from build123d import *

# Parameters (mm, degrees)
F0_R     = 4.5
F1_DEPTH = 8
F0_R_2   = 29
F0_R_3   = 27
F2_DEPTH = 4


with BuildPart() as f1:
    # F0 (on Front) → F1 (new body)
    with BuildSketch(Plane.XZ):
        Circle(F0_R)
    extrude(amount=F1_DEPTH)

    # F0 (on Front) → F2 (join)
    with BuildSketch(Plane.XZ):
        Circle(F0_R_2)
        Circle(F0_R_3, mode=Mode.SUBTRACT)
        Circle(F0_R_3)
        with BuildLine():
            ThreePointArc((4.3516162867, -22.646052221), (-0.1431680004, -25.9977219705), (-4.4156935051, -22.3669780097))
            Line((-4.4156935051, -22.3669780097), (0, -7.75))
            Line((0, -7.75), (4.3516162867, -22.646052221))
        make_face(mode=Mode.SUBTRACT)
        with BuildLine():
            ThreePointArc((-19.4040272759, -5.6313106345), (-17.9803864059, -4.3071155471), (-16.1592835692, -3.626064584))
            Line((-16.1592835692, -3.626064584), (-9.3891987076, -2.5182325158))
            ThreePointArc((-9.3891987076, -2.5182325158), (-7.4460025695, -2.583307283), (-5.6745435039, -3.3846678354))
            ThreePointArc((-5.6745435039, -3.3846678354), (-4.4349924254, -4.4349924254), (-3.3846678354, -5.6745435039))
            ThreePointArc((-3.3846678354, -5.6745435039), (-2.583307283, -7.4460025695), (-2.5182325158, -9.3891987076))
            Line((-2.5182325158, -9.3891987076), (-3.626064584, -16.1592835692))
            ThreePointArc((-3.626064584, -16.1592835692), (-4.3071155471, -17.9803864059), (-5.6313106345, -19.4040272759))
            ThreePointArc((-5.6313106345, -19.4040272759), (-18.3847763109, -18.3847763109), (-19.4040272759, -5.6313106345))
        make_face(mode=Mode.SUBTRACT)
        with BuildLine():
            Line((3.6418333236, -16.2556480886), (2.5157025337, -9.3737377061))
            ThreePointArc((2.5157025337, -9.3737377061), (2.5903516211, -7.3902488103), (3.4308544392, -5.5920953967))
            ThreePointArc((3.4308544392, -5.5920953967), (4.5023744658, -4.3693333532), (5.760194673, -3.3391923392))
            ThreePointArc((5.760194673, -3.3391923392), (7.5038582162, -2.5767129031), (9.4061289224, -2.5210029146))
            Line((9.4061289224, -2.5210029146), (16.060956923, -3.6099747692))
            ThreePointArc((16.060956923, -3.6099747692), (17.8462537904, -4.2691049062), (19.2559417587, -5.5475873168))
            ThreePointArc((19.2559417587, -5.5475873168), (18.450217913, -18.3171768004), (5.7146063745, -19.5483572234))
            ThreePointArc((5.7146063745, -19.5483572234), (4.344802068, -18.1118904301), (3.6418333236, -16.2556480886))
        make_face(mode=Mode.SUBTRACT)
        with BuildLine():
            ThreePointArc((-22.3669780097, -4.4156935051), (-26, 0), (-22.3669780097, 4.4156935051))
            Line((-22.3669780097, 4.4156935051), (-7.75, 0))
            Line((-7.75, 0), (-22.3669780097, -4.4156935051))
        make_face(mode=Mode.SUBTRACT)
        with BuildLine():
            Line((-9.3891987076, 2.5182325158), (-16.1592835692, 3.626064584))
            ThreePointArc((-16.1592835692, 3.626064584), (-17.9803864059, 4.3071155471), (-19.4040272759, 5.6313106345))
            ThreePointArc((-19.4040272759, 5.6313106345), (-18.3847763109, 18.3847763109), (-5.6313106345, 19.4040272759))
            ThreePointArc((-5.6313106345, 19.4040272759), (-4.3071155471, 17.9803864059), (-3.626064584, 16.1592835692))
            Line((-3.626064584, 16.1592835692), (-2.5182325158, 9.3891987076))
            ThreePointArc((-2.5182325158, 9.3891987076), (-2.583307283, 7.4460025695), (-3.3846678354, 5.6745435039))
            ThreePointArc((-3.3846678354, 5.6745435039), (-4.4349924254, 4.4349924254), (-5.6745435039, 3.3846678354))
            ThreePointArc((-5.6745435039, 3.3846678354), (-7.4460025695, 2.583307283), (-9.3891987076, 2.5182325158))
        make_face(mode=Mode.SUBTRACT)
        Circle(F0_R, mode=Mode.SUBTRACT)
        with BuildLine():
            Line((16.1592835692, 3.626064584), (9.3891987076, 2.5182325158))
            ThreePointArc((9.3891987076, 2.5182325158), (7.4460025695, 2.583307283), (5.6745435039, 3.3846678354))
            ThreePointArc((5.6745435039, 3.3846678354), (4.4349924254, 4.4349924254), (3.3846678354, 5.6745435039))
            ThreePointArc((3.3846678354, 5.6745435039), (2.583307283, 7.4460025695), (2.5182325158, 9.3891987076))
            Line((2.5182325158, 9.3891987076), (3.626064584, 16.1592835692))
            ThreePointArc((3.626064584, 16.1592835692), (4.3071155471, 17.9803864059), (5.6313106345, 19.4040272759))
            ThreePointArc((5.6313106345, 19.4040272759), (18.3847763109, 18.3847763109), (19.4040272759, 5.6313106345))
            ThreePointArc((19.4040272759, 5.6313106345), (17.9803864059, 4.3071155471), (16.1592835692, 3.626064584))
        make_face(mode=Mode.SUBTRACT)
        with BuildLine():
            ThreePointArc((22.3669780097, 4.4156935051), (26, 0), (22.3669780097, -4.4156935051))
            Line((22.3669780097, -4.4156935051), (7.75, 0))
            Line((7.75, 0), (14.262410288, 1.9673565762))
            Line((14.262410288, 1.9673565762), (22.3669780097, 4.4156935051))
        make_face(mode=Mode.SUBTRACT)
        with BuildLine():
            ThreePointArc((-4.4156935051, 22.3669780097), (0, 26), (4.4156935051, 22.3669780097))
            Line((4.4156935051, 22.3669780097), (0, 7.75))
            Line((0, 7.75), (-4.4156935051, 22.3669780097))
        make_face(mode=Mode.SUBTRACT)
    extrude(amount=F2_DEPTH)


solid = f1.part
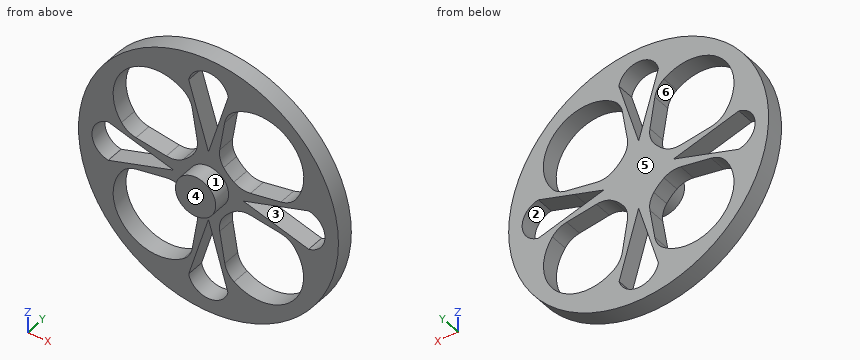
The listing builds one solid part. Answer for the finished solid, in the listing's coordinates (mm). Face numbers are marked on the shaded views. A direction names the side the tool comes from. Round coordinates to 2 decimals unless told otherwise and drop trailing zeros. Order: outer loops, then holes, each group sorted by start corner. A loop starts at its lowest first (then second) coordinate and runs counter-clockwise, first axis right, second up. Notation, with made-up numbers: (55.25, -30.5) - (61.25, -30.5) arc R21 cw to (61.25, -25.5) - close; hole circle Ø10 at (89.25, 6.25). An arc over 180 degrees is marked (long way). Write item = value, one per line. Start each with the question number.
1) For the marked faces 5 and 6, determine the directions among +Z, -Z, +X, -X, +Y, -Y from which every point of the face is accessible in a straight line to the end or side of a thin tool.
2) Section A-A, the plane x = 12 is taken. Write down the section's boundary in (y, z), plus the area to 3 significant figures.
3) Straight lines are drawn through the part: L1, parallel to X at y = -3, z = 9.5; L2, parallel to X at y = -1, z = 9; L3, parallel to Z at x = 4.5, y = -0.25. For each, find the intervals that lie inside material, in ascending order.
4) Given pin 1 (17.5 mm diameter, centred on x = 6, z = 13, fed in from -Y); pin 2 (3 mm diameter, centred on x = -6, y = -4.5, fed in from +Z), each flat-ended and moving along its own axis, determine where each tip first touches the part or whether it passes through.
5) For a pull along X with two mould halves and no side action, classify the marked faces 1, 2, 3 and 4 as released by +X, released by -X, zero draft, split by the parting line, or undercut.
6) Section D-D, the plane y = -2.75 is taken. Count the separate pieces of the cut face and the enclosed holes in it, plus the area to 3 significant figures.
7) Section B-B, the plane z = -7 is taken. Write down the section's boundary in (x, y).
8) Section C-C, the plane z = 18.5 is taken. Write down the section's boundary in (x, y).
Results list:
q1.face_5 = +Z, -Z, +X, -X, +Y
q1.face_6 = +Y, -Y
q2.outline = (-4, -26.4) - (0, -26.4) - (0, -21.3) - (-4, -21.3) - close; (-4, -2.95) - (0, -2.95) - (0, -1.28) - (-4, -1.28) - close; (-4, 1.28) - (0, 1.28) - (0, 2.95) - (-4, 2.95) - close; (-4, 21.26) - (0, 21.26) - (0, 26.4) - (-4, 26.4) - close
q2.area = 54.3 mm^2
q3.L1 = -27.4 to -21.09, -2.54 to -0.53, 0.53 to 2.54, 21.09 to 27.4
q3.L2 = -27.57 to -20.97, -2.47 to -0.38, 0.38 to 2.47, 20.97 to 27.57
q3.L3 = -28.65 to -18.34, -4.37 to 4.37, 18.27 to 28.65
q4.pin_1 = -4
q4.pin_2 = 28.64
q5.face_1 = split by the parting line
q5.face_2 = undercut
q5.face_3 = undercut
q5.face_4 = zero draft
q6.separate_pieces = 1
q6.enclosed_holes = 8
q6.area = 1,150 mm^2
q7.outline = (-28.14, -4) - (-20.23, -4) - (-20.23, 0) - (-28.14, 0) - close; (-2.71, -4) - (2.7, -4) - (2.7, 0) - (-2.71, 0) - close; (20.16, -4) - (28.14, -4) - (28.14, 0) - (20.16, 0) - close
q8.outline = (-22.33, -4) - (-18.27, -4) - (-18.27, 0) - (-22.33, 0) - close; (-4.68, -4) - (-3.25, -4) - (-3.25, 0) - (-4.68, 0) - close; (3.25, -4) - (4.68, -4) - (4.68, 0) - (3.25, 0) - close; (18.27, -4) - (22.33, -4) - (22.33, 0) - (18.27, 0) - close
